Input: part model. Units: mm. Frame: model coordinates. A direction names the side the tool comes from. Give positions to 0.01 mm unless a question says otherwise; leave off trailing zeros. Write each loop counter-clockwise with the first axis right and the second up, starting at its lowest first coordinate (ties: lowest second). Pieces come first, ordered by that corner, then holes. Notation, with made-up numbers: (60, -22.75) - (71, -22.75) arc R19 ccw to (71, 11.25) - close; hole circle Ø5 at (27, 47.5). An arc over 180 degrees is marked (long way). Use a Markdown table: item, result. Add a question column.
1. Mould query, pull axis Z, two halves, no side actions, for faces 4 (the flat face through (79, 12.83, 47)), 5 (the cylindrical face through (48.84, 6.12, 75.92)), 6 (the flat face through (79, 6, 95.37)). Classes: released by +Z, released by -Z, zero draft, split by the parting line, or undercut.
2. Section query D-D, the plane y = 5.5. Return loops of the section in (x, z) (3 decimals), plus the area to 3 significant figures.
3. Section query B-B, the plane z = 87.31. Return loops of the section in (x, y).
4. Section query C-C, the plane z = 48.5. Return loops of the section in (x, y).
5. Material intervals for probe 1 along Z at (x, y) = (152, 12); probe 2 along X at (y, z) = (1.5, 38.5); probe 3 along Z at (x, y) = (70, 11.5), sorted ascending.
6. Pin query (flat end, axial travel): pin 1 (3 mm diameter, centred on x = 134.5, z = 20.5, fed in from +Y); pin 2 (4 mm diameter, centred on y = 9, z = 46, fed in from +X); pin 3 (3 mm diameter, centred on x = 20, z = 6.5, fed in from -Y) (3 decimals). Return the tip coordinate at first contact, or that it passes through.
7. Section query A-A, the plane x = 50.46. Return loops of the section in (y, z).
8. Set-up query: faces 1 (the flat face through (148, 7, 35.81)), 2 (the flat face through (24, 9.83, 5)), 3 (the cylindrical face through (123.725, 1.628, 14.42)). Return all of +Z, -Z, +X, -X, +Y, -Y with unobstructed straight access to the full face (end or side cutting, diameter ignored); none if empty.
```python
from build123d import *

# Parameters (mm, degrees)
SKETCH1_W           = 160
SKETCH1_H           = 95.37
BOSS_EXTRUDE3_DEPTH = 12.83
HOLE1_D             = 18.97
SKETCH4_W           = 27.24
SKETCH4_H           = 28.56
CUT_EXTRUDE1_DEPTH  = 187.708451335
FILLET1_R           = 2.5
HOLE2_D             = 5.35
HOLE2_CBORE_D       = 10.65
HOLE2_CBORE_DEPTH   = 3
HOLE3_D             = 4.08
HOLE3_CSINK_D       = 5.5
HOLE3_CSINK_ANGLE   = 120
SKETCH10_R          = 9.525
CUT_EXTRUDE2_DEPTH  = 3.301941
SKETCH11_R          = 5.08
CUT_EXTRUDE3_DEPTH  = 3.175


with BuildPart() as part:
    # Sketch1 → Boss-Extrude3 (new body)
    with BuildSketch(Plane(origin=(0, 0, 0), x_dir=(1, 0, 0), z_dir=(0, 1, 0))):
        with Locations((80, -47.685)):
            Rectangle(SKETCH1_W, SKETCH1_H)
    extrude(amount=BOSS_EXTRUDE3_DEPTH)

    # Hole1 (through all)
    with Locations(Plane(origin=(0, 12.83, 0), x_dir=(-1, 0, 0), z_dir=(0, 1, 0))):
        with Locations((-32.885, 40.845), (-71.315, 40.845)):
            Hole(HOLE1_D / 2)

    # Sketch4 → Cut-Extrude1 (cut, through all)
    with BuildSketch(Plane(origin=(0, 12.83, 0), x_dir=(-1, 0, 0), z_dir=(0, 1, 0))):
        with Locations((-146.38, 50.09)):
            Rectangle(SKETCH4_W, SKETCH4_H)
    extrude(amount=-CUT_EXTRUDE1_DEPTH, mode=Mode.SUBTRACT)

    # Fillet1
    fillet1_edges = [part.edges().sort_by_distance(p)[0] for p in [
        (132.76, 6.415, 64.37),
        (132.76, 6.415, 35.81),
    ]]
    fillet(fillet1_edges, radius=FILLET1_R)

    # Hole2 (through all)
    with Locations(Plane(origin=(0, 12.83, 0), x_dir=(-1, 0, 0), z_dir=(0, 1, 0))):
        with Locations((-21.425, 6.17), (-132.175, 18.815)):
            CounterBoreHole(HOLE2_D / 2, HOLE2_CBORE_D / 2, HOLE2_CBORE_DEPTH)

    # Hole3 (through all)
    with Locations(Plane(origin=(0, 12.83, 0), x_dir=(-1, 0, 0), z_dir=(0, 1, 0))):
        with Locations((-50.46, 77.16), (-74.48, 87.31)):
            CounterSinkHole(HOLE3_D / 2, HOLE3_CSINK_D / 2, counter_sink_angle=HOLE3_CSINK_ANGLE)

    # Sketch10 → Cut-Extrude2 (cut)
    with BuildSketch(Plane.XZ):
        with Locations(Location((132.175, 18.815, 0), (0, 0, 270))):
            Circle(SKETCH10_R)
    extrude(amount=-CUT_EXTRUDE2_DEPTH, mode=Mode.SUBTRACT)

    # Sketch11 → Cut-Extrude3 (cut)
    with BuildSketch(Plane.XZ):
        with Locations(Location((21.425, 6.17, 0), (0, 0, 270))):
            Circle(SKETCH11_R)
    extrude(amount=-CUT_EXTRUDE3_DEPTH, mode=Mode.SUBTRACT)


solid = part.part
```
Result sheet:
| question | item | result |
|---|---|---|
| 1 | face 4 | zero draft |
| 1 | face 5 | undercut |
| 1 | face 6 | released by +Z |
| 2 | outline | (0, 0) - (160, 0) - (160, 35.81) - (135.26, 35.81) arc R2.5 cw to (132.76, 38.31) - (132.76, 61.87) arc R2.5 cw to (135.26, 64.37) - (160, 64.37) - (160, 95.37) - (0, 95.37) - close; hole circle Ø5.35 at (21.425, 6.17); hole circle Ø18.97 at (32.885, 40.845); hole circle Ø4.08 at (50.46, 77.16); hole circle Ø18.97 at (71.315, 40.845); hole circle Ø4.08 at (74.48, 87.31); hole circle Ø5.35 at (132.175, 18.815) |
| 2 | area | 13,800 mm² |
| 3 | outline | (0, 0) - (72.44, 0) - (72.44, 12.42) - (71.73, 12.83) - (0, 12.83) - close; (76.52, 0) - (160, 0) - (160, 12.83) - (77.23, 12.83) - (76.52, 12.42) - close |
| 4 | outline | (0, 0) - (27.28, 0) - (27.28, 12.83) - (0, 12.83) - close; (38.49, 0) - (65.71, 0) - (65.71, 12.83) - (38.49, 12.83) - close; (76.92, 0) - (132.76, 0) - (132.76, 12.83) - (76.92, 12.83) - close |
| 5 | probe 1 | z = 0 to 35.81, 64.37 to 95.37 |
| 5 | probe 2 | x = 0 to 23.69, 42.08 to 62.12, 80.51 to 132.76 |
| 5 | probe 3 | z = 0 to 31.45, 50.24 to 95.37 |
| 6 | pin 1 | stops at y = 9.83 |
| 6 | pin 2 | stops at x = 132.76 |
| 6 | pin 3 | stops at y = 3.175 |
| 7 | outline | (0, 0) - (12.83, 0) - (12.83, 74.41) - (12.42, 75.12) - (0, 75.12) - close; (0, 79.2) - (12.42, 79.2) - (12.83, 79.91) - (12.83, 95.37) - (0, 95.37) - close |
| 8 | face 1 | +X, +Y, -Y |
| 8 | face 2 | +Y |
| 8 | face 3 | -Y |
